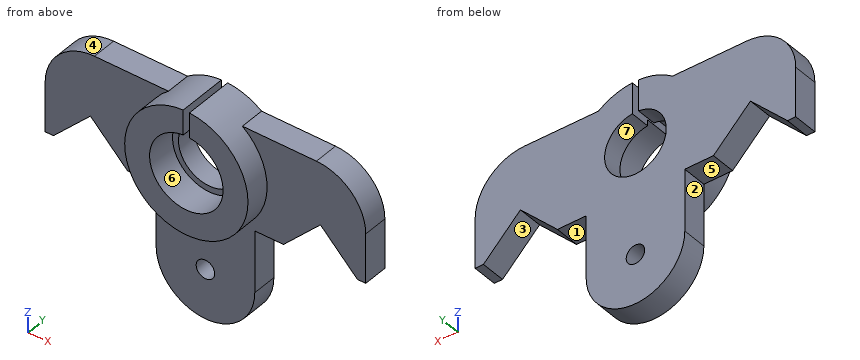
```python
from build123d import *

# Parameters (mm, degrees)
F0_R      = 15.875
F0_R_2    = 9.4615
F1_DEPTH  = 12.7
F3_DEPTH  = 6.35
F5_DEPTH  = 6.35
F7_R      = 12.7
F8_W      = 1.5875
F8_H      = 18.0220451
F9_DEPTH  = 12.701
F11_DEPTH = 5.08


with BuildPart() as f1:
    # F0 (on Front) → F1 (new body)
    with BuildSketch(Plane.XZ):
        Circle(F0_R)
        Circle(F0_R_2, mode=Mode.SUBTRACT)
    extrude(amount=F1_DEPTH)

    # F2 (on Front) → F3 (join)
    with BuildSketch(Plane.XZ):
        with BuildLine():
            Line((12.7, -9.525), (-12.7, -9.525))
            Line((-12.7, -9.525), (-12.7, -28.575))
            Line((-12.7, -28.575), (-2.38125, -28.575))
            ThreePointArc((-2.38125, -28.575), (0, -26.19375), (2.38125, -28.575))
            Line((2.38125, -28.575), (12.7, -28.575))
            Line((12.7, -28.575), (12.7, -9.525))
        make_face()
        with BuildLine():
            Line((-2.38125, -28.575), (-12.7, -28.575))
            ThreePointArc((-12.7, -28.575), (0, -41.275), (12.7, -28.575))
            Line((12.7, -28.575), (2.38125, -28.575))
            ThreePointArc((2.38125, -28.575), (0, -30.95625), (-2.38125, -28.575))
        make_face()
    extrude(amount=F3_DEPTH)

    # F4 (on Front) → F5 (join)
    with BuildSketch(Plane.XZ):
        Polygon((41.275, 12.7), (9.525, 12.7), (9.525, -12.7), (20.088640973, -12.7), (29.613640973, -3.175), (39.138640973, -12.7), (41.275, -12.7), align=None)
    extrude(amount=F5_DEPTH)

    # F6: F1 across plane


with BuildPart() as f1_1:
    add(f1.part)
    add(f1.part.mirror(Plane.YZ))

    # F7
    f7_edges = [f1_1.edges().sort_by_distance(p)[0] for p in [
        (41.275, -3.175, 12.7),
        (-41.275, -3.175, 12.7),
    ]]
    fillet(f7_edges, radius=F7_R)

    # F8 (on Front) → F9 (cut, through all)
    with BuildSketch(Plane.XZ):
        with Locations((0, 9.5910543679)):
            Rectangle(F8_W, F8_H)
    extrude(amount=F9_DEPTH, mode=Mode.SUBTRACT)

    # F10 (on Front) → F11 (join)
    with BuildSketch(Plane.XZ):
        with BuildLine():
            Line((-0.79375, 7.897712782), (-0.79375, 9.4281463283))
            ThreePointArc((-0.79375, 9.4281463283), (0, -9.4615), (0.79375, 9.4281463283))
            Line((0.79375, 9.4281463283), (0.79375, 7.897712782))
            ThreePointArc((0.79375, 7.897712782), (0, -7.9375), (-0.79375, 7.897712782))
        make_face()
    extrude(amount=F11_DEPTH)


solid = f1_1.part
```
The listing builds one solid part. Answer for the finished solid, in the listing's coordinates (mm). Face numbers are marked on the shaded views. A direction names the side the tool comes from. Give positions to 0.01 mm unless a question says otherwise; leave off trailing zeros. Order: outer loops, then holes, each group sorted by start corner. A loop starts at its lowest first (then second) coordinate and runs counter-clockwise, first axis right, second up. Notation, with made-up numbers: (-22, 28) - (-8, 28) arc R31 cw to (-8, 60) - close; hole circle Ø8 at (71, 11). An arc over 180 degrees is marked (long way). Use one line per item in the form item = value. Start each with the question number.
(1) For the marked faces 1, 2 and 3, determine the directions among +Z, -Z, +X, -X, +Y, -Y from which every point of the face is accessible in a straight line to the end or side of a thin tool.
(2) Flat-ended cylindrical pins translate along their axes: pin 1 Ø1.5 at (x, y) = (-24.5, -4.5) entering from +Z; pin 2 Ø4 at (x, y) = (27.5, -7) entering from -Z; pin 3 Ø5 at (x, y) = (-15.5, -4) entering from -Z. Find the tip coordinate at first contact, or state that the pin passes through.
(3) Consider line 1 (X direction, y = -8, z = 0) (1 decimal); line 2 (Z direction, x = 0, y = -3.55) (1 decimal); line 3 (X direction, y = -0.75, z = -4) (3 decimals). Determine where each line is inside the solid, lowest interval first. Write a range as from..to.
(4) A cutting plane is placed at C-C, the plane x = 6. Write down the section's boundary in (y, z), then the cut area to 3 significant figures.
(5) A cutting plane is placed at B-B, the plane z = 11.5. Write down the section's boundary in (x, y), then the cut area to 3 significant figures.
(6) The mould has two halves that part along Z. Classify the marked faces 4, 5, 6 and 7: released by +Z, released by -Z, zero draft, split by the parting line, or undercut.
Ans:
q1.face_1 = -Z, +X, +Y, -Y
q1.face_2 = -Z, -X, +Y, -Y
q1.face_3 = -Z, +Y, -Y
q2.pin_1 = 12.7
q2.pin_2 = -7.18
q2.pin_3 = -12.7
q3.line_1 = -15.9..-9.5, 9.5..15.9
q3.line_2 = -41.3..-31, -26.2..-7.9
q3.line_3 = -41.275..-30.439, -28.789..-6.856, 6.856..28.789, 30.439..41.275
q4.outline = (-12.7, -14.7) - (-6.35, -14.7) - (-6.35, -39.77) - (0, -39.77) - (0, -5.2) - (-5.08, -5.2) - (-5.08, -7.32) - (-12.7, -7.32) - close; (-12.7, 7.32) - (-5.08, 7.32) - (-5.08, 5.2) - (0, 5.2) - (0, 14.7) - (-12.7, 14.7) - close
q4.area = 368 mm^2
q5.outline = (-33.96, -6.35) - (-10.94, -6.35) - (-10.94, -12.7) - (-0.79, -12.7) - (-0.79, 0) - (-33.96, 0) - close; (0.79, -12.7) - (10.94, -12.7) - (10.94, -6.35) - (33.96, -6.35) - (33.96, 0) - (0.79, 0) - close
q5.area = 550 mm^2
q6.face_4 = released by +Z
q6.face_5 = released by -Z
q6.face_6 = undercut
q6.face_7 = undercut
